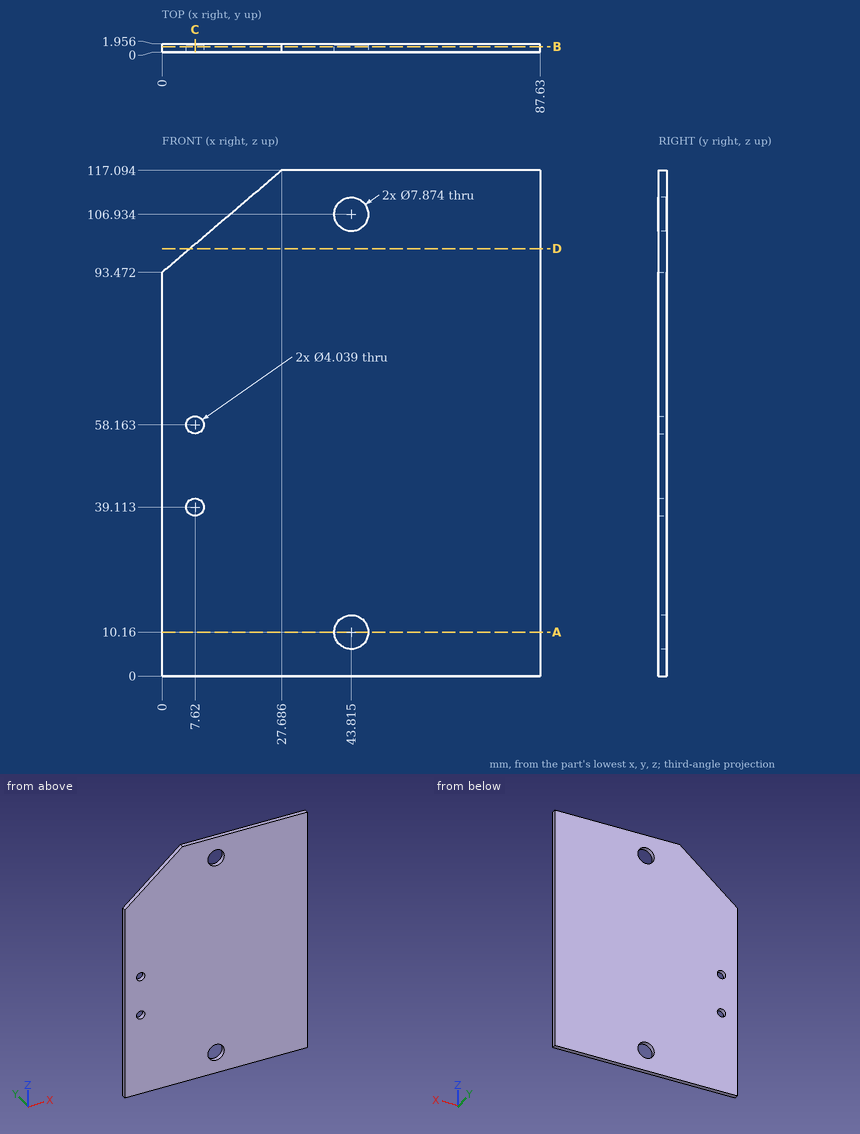
Check sheet for the drawn part. Datum: minimum x, y, z corner. Units: mm. Coordinates: 2 decimals unless noted, no trailing zeros. Order: outer loops, then holes, each group sorted by start corner. A loop starts at its lowest first (then second) coordinate and runs counter-clockwise, first axis right, second up. Notation, with made-up numbers: (79, 2) - (89, 2) arc R28 cw to (89, 24) - close; hole circle Ø1 at (1, -34). An arc over 180 degrees is marked (long way). Return JSON: item names as keys, results as strings.
(1) Section check A-A, the plane z = 10.16. Record the cut outline in (x, y) (1 decimal), and give its area (3 significant figures).
Filled sheet:
{"outline": "(0, 0) - (39.9, 0) - (39.9, 2) - (0, 2) - close; (47.8, 0) - (87.6, 0) - (87.6, 2) - (47.8, 2) - close", "area": "156 mm^2"}
(2) Section check B-B, the plane y = 1.35. Record the cut outline in (x, z) (1 decimal).
Filled sheet:
{"outline": "(0, 0) - (87.6, 0) - (87.6, 117.1) - (27.7, 117.1) - (0, 93.5) - close; hole circle Ø4 at (7.6, 39.1); hole circle Ø4 at (7.6, 58.2); hole circle Ø7.9 at (43.8, 10.2); hole circle Ø7.9 at (43.8, 106.9)"}
(3) Thickness scan on line 1 along Z through (x, y) = (7.62, 1.4) (1 decimal); line 2 along X through (y, z) = (1.65, 101.5); line 3 along Z through (x, y) = (18, 0.3). Record the ranges inside material, lowest first.
Filled sheet:
{"line 1": "z = 0 to 37.1, 41.1 to 56.1, 60.2 to 100", "line 2": "x = 9.41 to 87.63", "line 3": "z = 0 to 108.83"}
(4) Go/stop test with a flat-tipped pin: pin 1 (8 mm diameter, centred on x = 64.5, z = 24, fed in from -Y). Record where the tip stops, or that it passes through.
Filled sheet:
{"pin 1": "stops at y = 0"}
(5) Section check D-D, the plane z = 99. Record the cut outline in (x, y) (1 decimal).
Filled sheet:
{"outline": "(6.5, 0) - (87.6, 0) - (87.6, 2) - (6.5, 2) - close"}
(6) Section check C-C, the plane x = 7.62. Record the cut outline in (y, z) (1 decimal).
Filled sheet:
{"outline": "(0, 0) - (2, 0) - (2, 37.1) - (0, 37.1) - close; (0, 41.1) - (2, 41.1) - (2, 56.1) - (0, 56.1) - close; (0, 60.2) - (2, 60.2) - (2, 100) - (0, 100) - close"}
